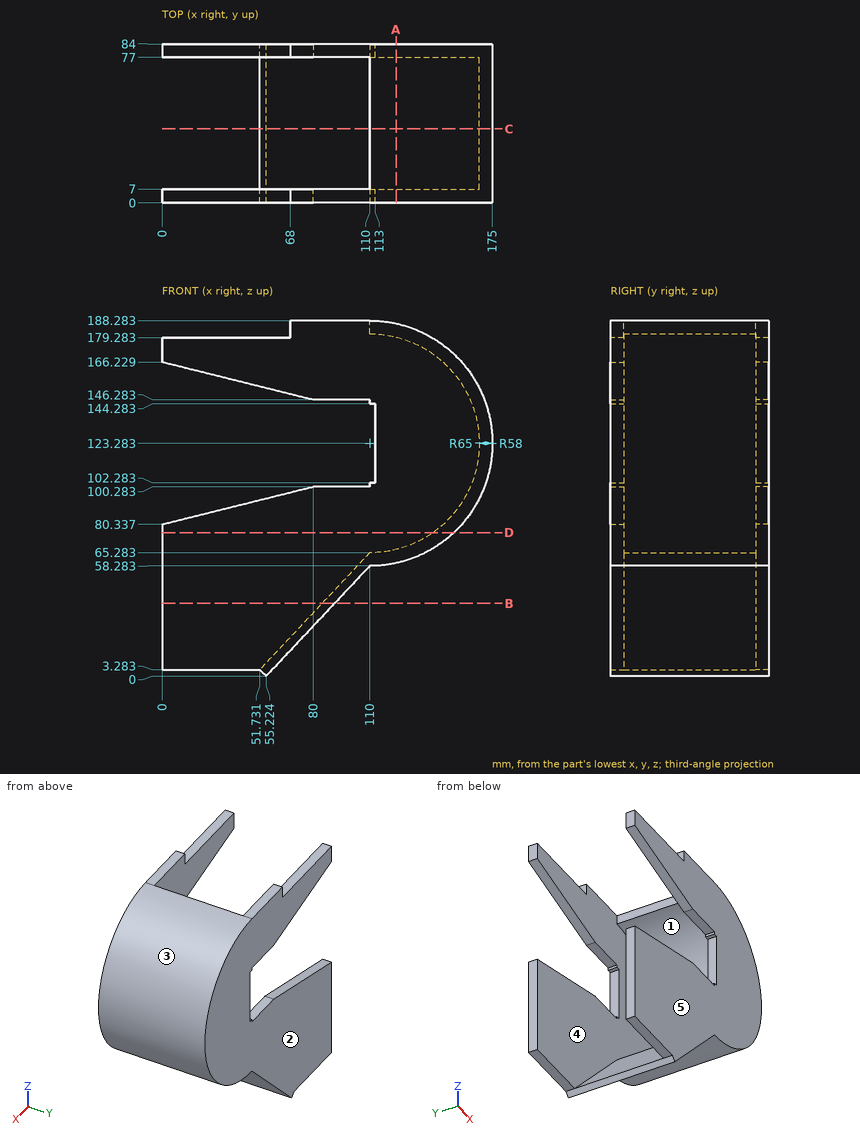
The figure shows three views and two pictorial views of one solid part (mm, origin at its lowest corner). Answer the questions. A direction names the side the tool comes from. Round coordinates to 2 decimals unless told otherwise and drop trailing zeros. Order: outer loops, then holes, each group sorted by start corner. A loop starts at its lowest first (then second) coordinate and runs counter-clockwise, first axis right, second up. Notation, with made-up numbers: M 58,-0.75 L 90,-0.75 A25 ccw 90,29.25 Z; hole C 41.25,74 d10. An arc over 180 degrees is marked long. Answer in a Markdown table with one row per item. Add a question column.
1) Which of the six approach directions +Z, -Z, +X, -X, +Y, -Y give full straight-line access (tool end or side, diameter ignored) to the marked faces 1 and 2?
2) The part is cut by section D-D on z = 76. Determine the outline of the cut face in (x, y).
3) The part is cut by section C-C on y = 39. Determine the outline of the cut face in (x, z) (1 decimal).
4) Consider line 1 along Y through (x, z) = (124, 99.5); line 2 along Z through (x, y) = (151.5, 16) (1 decimal); line 3 along Z through (x, y) = (122, 70) (1 decimal). Determine where each line is inside the solid, lowest interval first. Write a range as from..to.
5) The part is cut by section A-A on x = 124. Determine the outline of the cut face in (y, z), plus the area to 3 significant figures.
6) The part is cut by section B-B on z = 38.5. Determine the outline of the cut face in (x, y), plus the area to 3 significant figures.
7) Flat-ended cylindrical pins translate along their axes: pin 1 Ø2 at (x, y) = (90.5, 81.5) entering from -Z; pin 2 Ø2 at (y, z) = (48, 168.5) entering from +X; pin 3 Ø5.5 at (y, z) = (79.5, 183) entering from -X. Find the tip coordinate at first contact, or state that the pin passes through.
8) Determine the mould class of the marked faces 3, 4 and 5 for opening direction Z: pulls with the +Z half, pulls with the -Z half, needs draft (parallel to the pull), parting line crosses it, or undercut.
Findings below:
| question | item | result |
|---|---|---|
| 1 | face 1 | -X |
| 1 | face 2 | +Z, -Z, +X, -X, +Y |
| 2 | outline | M 0,0 L 154.6,0 L 154.6,84 L 0,84 L 0,77 L 143.59,77 L 143.59,7 L 0,7 Z |
| 3 | outline | M 51.7,3.3 L 55.2,0 L 110,58.3 A65 ccw 110,188.3 L 110,181.3 A58 cw 110,65.3 Z |
| 4 | line 1 | y = 0..7, 77..84 |
| 4 | line 2 | z = 73.3..82.8, 163.8..173.3 |
| 4 | line 3 | z = 59.4..66.5, 180..187.2 |
| 5 | outline | M 0,59.81 L 84,59.81 L 84,186.76 L 0,186.76 Z; hole M 7,67 L 77,67 L 77,179.57 L 7,179.57 Z |
| 5 | area | 2,780 mm² |
| 6 | outline | M 0,0 L 91.41,0 L 91.41,84 L 0,84 L 0,77 L 84.83,77 L 84.83,7 L 0,7 Z |
| 6 | area | 1,740 mm² |
| 7 | pin 1 | stops at z = 36.47 |
| 7 | pin 2 | stops at x = 157.64 |
| 7 | pin 3 | stops at x = 68 |
| 8 | face 3 | parting line crosses it |
| 8 | face 4 | undercut |
| 8 | face 5 | needs draft |
